Part model, mm, in its own coordinate system. Face numbers are marked on the shaded views. A direction names the side the tool comes from. Round coordinates to 2 decimals unless told otherwise and drop trailing zeros. Order: outer loops, then holes, each group sorted by start corner. A loop starts at its lowest first (then second) coordinate and runs counter-clockwise, first axis right, second up. Notation, with made-up numbers: (77, 53) - (91, 53) arc R7 ccw to (91, 62) - close; hole circle Ø6 at (-4.75, 26.25). An arc over 180 degrees is marked (long way). Return JSON: item names as keys, results as strings. Group by question number.
Item 1: Probe probe 1 along X at (y, z) = (1, 2); probe 2 along X at (y, z) = (6.75, 8.75); probe 3 along X at (y, z) = (-1, 6.25). List the from-to ranges inside material, lowest first.
Item 2: Drop flat-ended pins along their axis: pin 1 (3 mm diameter, centred on x = 4.5, z = 8, fed in from +Y); pin 2 (5.5 mm diameter, centred on y = 4, z = 3, fed in from -X); pin 3 (1.7 mm diameter, centred on y = 5.5, z = 6, fed in from +X); pin 4 (1.7 mm diameter, centred on y = 4.5, z = 4, fed in from -X). Give the stop position or say it passes through.
Item 3: Saw through at B-B on z = 1.5. List the corners of the cut face in (x, y), and give its area (3 significant figures).
Item 4: Tool access for the marked faces 1 and 2: list every direction of +Z, -Z, +X, -X, +Y, -Y with a clear straight run to the whole face (end or side of a thin tool).
Item 5: Saw through at A-A on x = 11. List the corners of the cut face in (y, z).
Item 6: Saw through at C-C on x = -15. List the corners of the cut face in (y, z), and give its area (3 significant figures).
Item 7: Saw through at D-D on y = 3.5. State how many separate pieces and enclosed holes the cut face has, and give its area (3 significant figures).
```python
from build123d import *

# Parameters (mm, degrees)
BOSS_EXTRUDE1_DEPTH = 10
SKETCH2_R           = 1.6
CUT_EXTRUDE1_DEPTH  = 44.1
CUT_EXTRUDE2_DEPTH  = 2
CUT_EXTRUDE3_DEPTH  = 2.5
SKETCH6_W           = 20
SKETCH6_H           = 6
CUT_EXTRUDE4_DEPTH  = 11


with BuildPart() as part:
    # Sketch1 → Boss-Extrude1 (new body)
    with BuildSketch(Plane.XY):
        with BuildLine():
            Line((-21.55, 7.2), (-17.55, 7.2))
            Line((-17.55, 7.2), (-17.55, 0.2))
            ThreePointArc((-17.55, 0.2), (-15, -2.35), (-12.45, 0.2))
            Line((-12.45, 0.2), (-12.45, 7.2))
            Line((-12.45, 7.2), (12.45, 7.2))
            Line((12.45, 7.2), (12.45, 0.2))
            ThreePointArc((12.45, 0.2), (15, -2.35), (17.55, 0.2))
            Line((17.55, 0.2), (17.55, 7.2))
            Line((17.55, 7.2), (21.55, 7.2))
            Line((21.55, 7.2), (21.55, -10.574417152))
            Line((21.55, -10.574417152), (-21.55, -10.574417152))
            Line((-21.55, -10.574417152), (-21.55, 7.2))
        make_face()
    extrude(amount=BOSS_EXTRUDE1_DEPTH)

    # Sketch2 → Cut-Extrude1 (cut, through all)
    with BuildSketch(Plane(origin=(21.55, 0, 0), x_dir=(0, 0, -1), z_dir=(1, 0, 0))):
        with Locations((-5.28643622, 4.4)):
            Circle(SKETCH2_R)
    extrude(amount=-CUT_EXTRUDE1_DEPTH, mode=Mode.SUBTRACT)

    # Sketch3 → Cut-Extrude2 (cut)
    with BuildSketch(Plane(origin=(21.55, 0, 0), x_dir=(0, 0, -1), z_dir=(1, 0, 0))):
        with BuildLine():
            Line((-8.28643622, 7.2), (-2.28643622, 7.2))
            Line((-2.28643622, 7.2), (-2.28643622, 4.4))
            ThreePointArc((-2.28643622, 4.4), (-5.28643622, 1.4), (-8.28643622, 4.4))
            Line((-8.28643622, 4.4), (-8.28643622, 7.2))
        make_face()
    extrude(amount=-CUT_EXTRUDE2_DEPTH, mode=Mode.SUBTRACT)

    # Sketch4 → Cut-Extrude3 (cut)
    with BuildSketch(Plane.ZY.offset(21.55)):
        Polygon((8.519597728, 4.4), (6.903016974, 7.2), (3.669855466, 7.2), (2.053274713, 4.4), (3.669855466, 1.6), (6.903016974, 1.6), align=None)
    extrude(amount=-CUT_EXTRUDE3_DEPTH, mode=Mode.SUBTRACT)

    # Sketch6 → Cut-Extrude4 (cut, through all)
    with BuildSketch(Plane.XY.offset(10)):
        with Locations((0, 4.2)):
            Rectangle(SKETCH6_W, SKETCH6_H)
    extrude(amount=-CUT_EXTRUDE4_DEPTH, mode=Mode.SUBTRACT)


solid = part.part
```
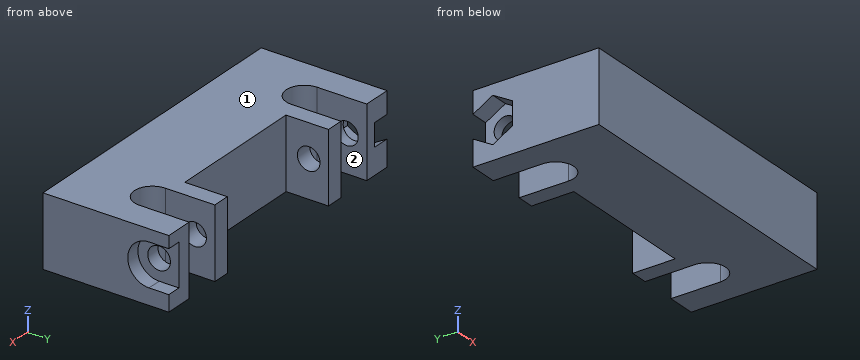
Filled in:
{
 "1": {"probe 1": "x = -21.55 to -17.55, -12.45 to 12.45, 17.55 to 21.55", "probe 2": "x = -21.55 to -17.55, -12.45 to -10, 10 to 12.45, 17.55 to 21.55", "probe 3": "x = -21.55 to -17.25, -12.75 to 12.75, 17.25 to 21.55"},
 "2": {"pin 1": "stops at y = 1.2", "pin 2": "stops at x = -21.55", "pin 3": "stops at x = 19.55", "pin 4": "stops at x = -19.05"},
 "3": {"outline": "(-21.55, -10.57) - (21.55, -10.57) - (21.55, 7.2) - (17.55, 7.2) - (17.55, 0.2) arc R2.55 cw to (12.45, 0.2) - (12.45, 7.2) - (10, 7.2) - (10, 1.2) - (-10, 1.2) - (-10, 7.2) - (-12.45, 7.2) - (-12.45, 0.2) arc R2.55 cw to (-17.55, 0.2) - (-17.55, 7.2) - (-21.55, 7.2) - close", "area": "554 mm^2"},
 "4": {"face 1": "+Z, +X, -X, +Y, -Y", "face 2": "+Z, -Z, +Y"},
 "5": {"outline": "(-10.57, 0) - (7.2, 0) - (7.2, 10) - (-10.57, 10) - close; hole circle Ø3.2 at (4.4, 5.29)"},
 "6": {"outline": "(-10.57, 0) - (-2.35, 0) - (-2.35, 10) - (-10.57, 10) - close", "area": "82.2 mm^2"},
 "7": {"separate pieces": "8", "enclosed holes": "0", "area": "81.8 mm^2"}
}
